from build123d import *

# Parameters (mm, degrees)
SKETCH076_W             = 40
SKETCH076_H             = 15
PAD026_DEPTH            = 50
SKETCH078_W             = 40
SKETCH078_H             = 24
PAD027_DEPTH            = 40
SKETCH079_W             = 32
SKETCH079_H             = 16
POCKET046_DEPTH         = 40.001
FILLET010_R             = 3.5
BODY011_ROLL_ANGLE      = 90
BODY011_PLACEMENT_ANGLE = 180
SKETCH057_W             = 120
SKETCH057_H             = 40
PAD021_DEPTH            = 15
SKETCH058_R             = 15
POCKET034_DEPTH         = 5
POCKET035_DEPTH         = 5
SKETCH060_R             = 7.7
POCKET036_DEPTH         = 15.001


with BuildPart() as obj1:
    # Sketch076 → Pad026 (new body)
    with BuildSketch(Plane.YZ):
        with Locations((20, 7.5)):
            Rectangle(SKETCH076_W, SKETCH076_H)
    extrude(amount=PAD026_DEPTH)

    # Sketch078 → Pad027 (join)
    with BuildSketch(Plane.XZ):
        with Locations((30, -12)):
            Rectangle(SKETCH078_W, SKETCH078_H)
    extrude(amount=-PAD027_DEPTH)

    # Sketch079 → Pocket046 (cut, through all)
    with BuildSketch(Plane.XZ):
        with Locations((26, -8)):
            Rectangle(SKETCH079_W, SKETCH079_H)
    extrude(amount=-POCKET046_DEPTH, mode=Mode.SUBTRACT)

    # Fillet010
    fillet010_edges = [obj1.edges().sort_by_distance(p)[0] for p in [
        (10, 20, -24),
        (10, 0, -20),
        (26, 0, -16),
        (30, 0, -24),
        (10, 20, -16),
        (10, 40, -20),
        (30, 40, -24),
        (26, 40, -16),
    ]]
    fillet(fillet010_edges, radius=FILLET010_R)


with BuildPart() as obj1_1:
    # Body011 roll: moved
    add(obj1.part.rotate(Axis((0, 0, 0), (1, 0, 0)), BODY011_ROLL_ANGLE))


with BuildPart() as obj1_2:
    # Body011 placement: moved
    add(obj1_1.part.moved(Location((-71, -15, -20))).rotate(Axis((-71, -15, -20), (0, 0, 1)), BODY011_PLACEMENT_ANGLE))


with BuildPart() as bracket_b:
    # Sketch057 → Pad021 (new body)
    with BuildSketch(Plane.XZ):
        with Locations((-12, 0)):
            Rectangle(SKETCH057_W, SKETCH057_H)
    extrude(amount=PAD021_DEPTH)

    # Sketch058 (on Face6 of Pad021) → Pocket034 (cut)
    with BuildSketch(Plane.XZ.offset(15)):
        Circle(SKETCH058_R)
    extrude(amount=-POCKET034_DEPTH, mode=Mode.SUBTRACT)

    # Sketch059 → Pocket035 (cut)
    with BuildSketch(Plane.XZ):
        Polygon((9.608347, 3.979908), (3.979908, 9.608347), (-3.979908, 9.608347), (-9.608347, 3.979908), (-9.608347, -3.979908), (-3.979908, -9.608347), (3.979908, -9.608347), (9.608347, -3.979908), align=None)
    extrude(amount=POCKET035_DEPTH, mode=Mode.SUBTRACT)

    # Sketch060 → Pocket036 (cut, through all)
    with BuildSketch(Plane.XZ):
        Circle(SKETCH060_R)
    extrude(amount=POCKET036_DEPTH, mode=Mode.SUBTRACT)

    # Boolean: union obj1
    add(obj1_2.part)


solid = bracket_b.part
The model under review builds one solid part; all positions refer to its coordinate system, in mm. A direction names the side the tool comes from. Round coordinates to 2 decimals unless told otherwise and drop trailing zeros. Order: outer loops, then holes, each group sorted by start corner. A loop starts at its lowest first (then second) coordinate and runs counter-clockwise, first axis right, second up. Notation, with made-up numbers: (44.25, 73) - (60.25, 73) arc R10 ccw to (60.25, 82) - close; hole circle Ø5 at (33, 37.5). An arc over 180 degrees is marked (long way). Use one line per item in the form item = value.
Q1. Add section B-B on x = -91.5. Give the boundary of the cut face in (y, z).
Response values:
outline = (-39, -16.5) arc R3.5 ccw to (-35.5, -20) - (-34.5, -20) arc R3.5 ccw to (-31, -16.5) - (-31, 16.5) arc R3.5 ccw to (-34.5, 20) - (-35.5, 20) arc R3.5 ccw to (-39, 16.5) - close; (-15, -20) - (0, -20) - (0, 20) - (-15, 20) - close
Q2. Tool access review of faces 5 (the cylindrical face through (-82, -34.99, -18.95)), 6 (the flat face through (-121, -20, 0)), 7 (the cylindrical face through (-14.985, -12.535, 0.66)), 8 (the flat face through (0, -2, -9.608)), 9 (the cylindrical face through (-82, -32.05, 0.23)): name each direction out of +Z, -Z, +X, -X, +Y, -Y from which nothing blocks a thin tool from reaching the whole face with its end or side.
Response values:
face_5 = -Z, +X, -Y
face_6 = +Z, -Z, -X, +Y, -Y
face_7 = -Y
face_8 = +Y
face_9 = +Z, -Z, +X
Q3. Mouldability with a two-part tool opening along Z and no side actions: class faces 1 (the flat face through (6.755, -2.465, -6.834)), 2 (the flat face through (-35, -10, -20)), 3 (the flat face through (-99, -31, 0)), 4 (the cylindrical face through (-103.01, -38, 18.95)) as pulls with the +Z half, pulls with the -Z half, needs draft (parallel to the pull), parting line crosses it, or undercut.
Response values:
face_1 = undercut
face_2 = pulls with the -Z half
face_3 = needs draft
face_4 = pulls with the +Z half
Q4. Add section D-D on x = 23. Give the boundary of the cut face in (y, z), then the cut area to 3 significant figures.
Response values:
outline = (-15, -20) - (0, -20) - (0, 20) - (-15, 20) - close
area = 600 mm^2
Q5. Clearance check with flat-ended pins moving along their axes: P1, Ø9, axis at x = -6, z = 1.5, coming from the -Y side; P2, Ø12, axis at x = -8, z = -1, coming from the +Y side; P3, Ø15.5, axis at y = -27.5, z = 8, coming from the +X side. State where each tip first meets the part, or that it passes through.
Response values:
P1 = -10
P2 = 0
P3 = -81
Q6. Add section C-C on z = 13. Give the boundary of the cut face in (x, y), then the cut area to 3 significant figures.
Response values:
outline = (-121, -39) - (-84.5, -39) arc R3.5 ccw to (-81, -35.5) - (-81, -34.5) arc R3.5 ccw to (-84.5, -31) - (-113, -31) - (-113, -15) - (-7.48, -15) - (-7.48, -10) - (7.48, -10) - (7.48, -15) - (48, -15) - (48, 0) - (-121, 0) - close
area = 2,900 mm^2
Q7. To check wall thickness, follow line 1 (Z direction, x = 0, y = -8.6); line 2 (X direction, y = -1.5, z = -0.5); line 3 (Y direction, x = -0.5, z = 11.5). State the ranges of each line that lie inside material, in increasing order.
Response values:
line_1 = -20 to -7.7, 7.7 to 20
line_2 = -121 to -9.61, 9.61 to 48
line_3 = -10 to 0
Q8. Add section A-A on x = 0. Give the boundary of the cut face in (y, z).
Response values:
outline = (-15, -20) - (0, -20) - (0, -9.61) - (-5, -9.61) - (-5, -7.7) - (-10, -7.7) - (-10, -15) - (-15, -15) - close; (-15, 15) - (-10, 15) - (-10, 7.7) - (-5, 7.7) - (-5, 9.61) - (0, 9.61) - (0, 20) - (-15, 20) - close
